Could you check a few things on this model? Use its own coordinates, in mm. Coordinates: 2 decimals unless noted, no trailing zeros. Order: outer loops, then holes, each group sorted by start corner. A loop starts at its lowest first (then second) coordinate and runs counter-clockwise, first axis right, second up. Notation, with made-up numbers: (-7.5, 85) -> (50.5, 85) arc R26 ccw to (50.5, 102) -> close; hole circle Ø4 at (76, 29). An arc over 180 degrees is marked (long way). Use a Markdown table: item, result. Add a question column.
1) If we section it at B-B (z = 2): Write out the boundary of the cut face in (x, y).
2) If we section it at A-A (x = 0): Write out the boundary of the cut face in (y, z).
3) If I drill on L1, parallel to X at y = -12.75, z = 87; L2, parallel to Z at x = -14, y = -1.25; L3, parallel to Z at x = 175.5, y = -6, over which ranges is the centre line in solid material (lowest first)? Write a range as [from, to].
4) If we section it at D-D (y = -10.25): Give the number of separate pieces and of enclosed holes in the cut face, plus the area to 3 significant figures.
5) If we section it at C-C (x = -64): Write out the boundary of the cut face in (y, z), plus the area to 3 significant figures.
6) Will these pins go through, and if not, where does the flat tip stop? pin 1 Ø7 at (y, z) = (-2.5, 135) entering from -X; pin 2 Ø1.9 at (x, y) = (39.5, -2.5) entering from +Z; pin 3 Ø3 at (y, z) = (-2, -88) entering from +X.
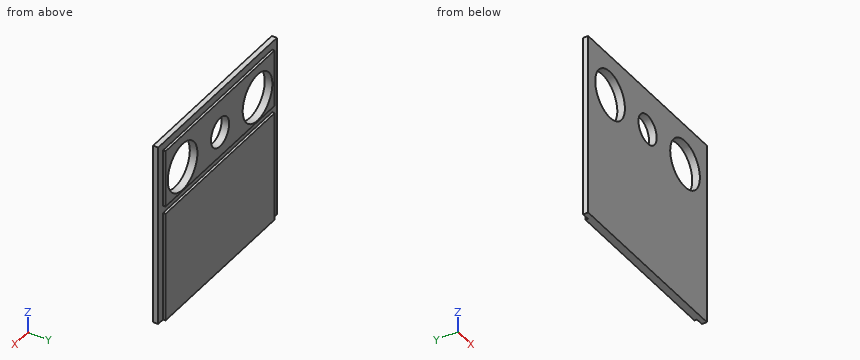
```python
from build123d import *

# Parameters (mm, degrees)
F0_W     = 482.6
F0_H     = 464.185
F1_DEPTH = 19.304
F3_D     = 73.914
F4_D     = 120.65
F5_W     = 19.304
F5_H     = 19.304
F5_W_2   = 443.992
F5_H_2   = 145.415
F5_H_3   = 280.162
F6_DEPTH = 6.35


with BuildPart() as f1:
    # F0 (on Front) → F1 (new body)
    with BuildSketch(Plane.XZ):
        Rectangle(F0_W, F0_H)
    extrude(amount=F1_DEPTH)

    # F3 (through all)
    with Locations(Plane.XZ.offset(19.304)):
        with Locations((0, 130.4925)):
            Hole(F3_D / 2)

    # F4 (through all)
    with Locations(Plane.XZ.offset(19.304)):
        with Locations((-152.444478, 130.4925), (152.444478, 130.4925)):
            Hole(F4_D / 2)

    # F5 (on face) → F6 (cut)
    with BuildSketch(Plane(origin=(0, 0, 0), x_dir=(-1, 0, 0), z_dir=(0, 1, 0))):
        with Locations((-231.648, 222.4405)):
            Rectangle(F5_W, F5_H)
        with Locations((0, 222.4405)):
            Rectangle(F5_W_2, F5_H)
        with Locations((-231.648, 140.081)):
            Rectangle(F5_W, F5_H_2)
        with Locations((231.648, 222.4405)):
            Rectangle(F5_W, F5_H)
        with Locations((-231.648, 57.7215)):
            Rectangle(F5_W, F5_H)
        with Locations((0, 57.7215)):
            Rectangle(F5_W_2, F5_H)
        with Locations((231.648, 140.081)):
            Rectangle(F5_W, F5_H_2)
        with Locations((-231.648, -92.0115)):
            Rectangle(F5_W, F5_H_3)
        with Locations((231.648, 57.7215)):
            Rectangle(F5_W, F5_H)
        with Locations((231.648, -92.0115)):
            Rectangle(F5_W, F5_H_3)
    extrude(amount=-F6_DEPTH, mode=Mode.SUBTRACT)


solid = f1.part
```
Answer sheet:
| question | item | result |
|---|---|---|
| 1 | outline | (-241.3, -19.3) -> (241.3, -19.3) -> (241.3, -6.35) -> (222, -6.35) -> (222, 0) -> (-222, 0) -> (-222, -6.35) -> (-241.3, -6.35) -> close |
| 2 | outline | (-19.3, -232.09) -> (0, -232.09) -> (0, 48.07) -> (-6.35, 48.07) -> (-6.35, 67.37) -> (0, 67.37) -> (0, 93.54) -> (-19.3, 93.54) -> close; (-19.3, 167.45) -> (0, 167.45) -> (0, 212.79) -> (-6.35, 212.79) -> (-6.35, 232.09) -> (-19.3, 232.09) -> close |
| 3 | L1 | [-241.3, -194.25], [-110.64, 110.64], [194.25, 241.3] |
| 3 | L2 | [-232.09, 48.07], [67.37, 96.29], [164.7, 212.79] |
| 3 | L3 | [-232.09, 48.07], [67.37, 74.75], [186.24, 212.79] |
| 4 | separate pieces | 1 |
| 4 | enclosed holes | 3 |
| 4 | area | 197,000 mm2 |
| 5 | outline | (-19.3, -232.09) -> (0, -232.09) -> (0, 48.07) -> (-6.35, 48.07) -> (-6.35, 67.37) -> (0, 67.37) -> (0, 212.79) -> (-6.35, 212.79) -> (-6.35, 232.09) -> (-19.3, 232.09) -> close |
| 5 | area | 8,720 mm2 |
| 6 | pin 1 | x = -222 |
| 6 | pin 2 | z = 212.79 |
| 6 | pin 3 | x = 222 |
